Geometry check sheet. Reference: the model listing, model coordinates, mm. A direction names the side the tool comes from. Coordinates: 2 decimals unless noted, no trailing zeros. Order: outer loops, then holes, each group sorted by start corner. A loop starts at its lowest first (then second) coordinate and runs counter-clockwise, first axis right, second up. Notation, with made-up numbers: M 39.5,31 L 93.5,31 A31 ccw 93.5,56 Z; hole C 22,33.25 d7. An arc over 180 degrees is marked long. One line per item, written item: value. Start each with the question number.
1) Thickness scan on L1, parallel to X at y = 59, z = 2.5; L2, parallel to X at y = 49, z = 17; L3, parallel to X at y = -18, z = 11.5. Record the ranges inside material, lowest first. Write a range as from..to.
2) Sectioned sample at B-B, the plane x = -41.5. Enter the section's corners in (y, z), then the cut area to 3 significant figures.
3) Access from +Z, -Z, +X, -X, +Y, -Y to the whole of each face (thin tool, end or side, straight path). Record for faces 4 (the flat face through (-35.057, -29.095, 12.522)), 5 (the flat face through (53.315, 29.328, 12.522)).
4) Sectioned sample at D-D, the plane y = 75. Enter the section's corners in (x, z).
5) Go/stop test with flat-tipped pins: P1, Ø3, axis at x = -68, z = 13, coming from the +Y side; P2, Ø10, axis at y = 33.5, z = 3, coming from the +X side; P3, Ø3, axis at x = 53.5, z = 10.5, coming from the -Y side. Record where each tip stops, or that it passes through.
6) Sectioned sample at C-C, the plane z = 21.25. Enter the section's corners in (x, y), then the cut area to 3 significant figures.
7) Sectioned sample at A-A, the plane y = 35.5. Enter the section's corners in (x, z), then the cut area to 3 significant figures.
8) Draft check along Y on faces 1 (the flat face through (-25, -9, 0)), 2 (the flat face through (-52.056, 31.509, 12.522)), 3 (the flat face through (42.725, -15.813, 12.522)). Enter one of: pulls with the +Y half, pulls with the -Y half, needs draft (parallel to the pull), parting line crosses it, or undercut.
```python
from build123d import *

# Parameters (mm, degrees)
F1_DEPTH = 25.4


with BuildPart() as f1:
    # F0 (on Top) → F1 (new body)
    with BuildSketch(Plane.XY):
        Polygon((-105.146734, -61.205373), (105.578775, -60.457056), (-0.432041, 121.66243), align=None)
        Polygon((62.332636, -31.189396), (66.488145, -38.386948), (58.177127, -38.386948), (49.866109, -38.386948), (33.244072, -38.386948), (0, -38.386948), (-33.244072, -38.386948), (-49.866109, -38.386948), (-58.177127, -38.386948), (-66.488145, -38.386948), (-62.332636, -31.189396), (-58.177127, -23.991843), (-49.866109, -9.596737), (-33.244072, 19.193474), (-16.622036, 47.983686), (-8.311018, 62.378791), (-4.155509, 69.576344), (0, 76.773897), (4.155509, 69.576344), (8.311018, 62.378791), (16.622036, 47.983686), (33.244072, 19.193474), (49.866109, -9.596737), (58.177127, -23.991843), align=None, mode=Mode.SUBTRACT)
        Polygon((-58.177127, -38.386948), (-11.280757, -19.538844), (-22.561514, 0), (-62.332636, -31.189396), (-66.488145, -38.386948), align=None)
        Polygon((0, 19.538844), (11.280757, 19.538844), (4.155509, 69.576344), (0, 76.773897), (-4.155509, 69.576344), (-11.280757, 19.538844), align=None)
        Polygon((58.177127, -38.386948), (66.488145, -38.386948), (62.332636, -31.189396), (22.561514, 0), (11.280757, -19.538844), align=None)
    extrude(amount=F1_DEPTH)


solid = f1.part
```
Final values:
1. L1: x = -36.31..-10.26, -5.66..5.66, 10.26..36.04
1. L2: x = -42.04..-16.04, -7.09..7.09, 16.04..41.86
1. L3: x = -80.41..-54.72, -45.51..-12.17, 12.17..45.51, 54.72..80.86
2. outline: M -60.98,0 L -38.39,0 L -38.39,25.4 L -60.98,25.4 Z; M -31.68,0 L -14.85,0 L -14.85,25.4 L -31.68,25.4 Z; M 4.89,0 L 49.94,0 L 49.94,25.4 L 4.89,25.4 Z
2. area: 2,150 mm^2
3. face 4: +Z, -Z
3. face 5: +Z, -Z, +X, +Y
4. outline: M -27.15,0 L 26.73,0 L 26.73,25.4 L -27.15,25.4 Z
5. P1: stops at y = 6.29
5. P2: stops at x = 53.8
5. P3: stops at y = -60.65
6. outline: M -105.15,-61.21 L 105.58,-60.46 L -0.43,121.66 Z; hole M -62.33,-31.19 L -22.56,0 L -11.28,-19.54 L -58.18,-38.39 L 58.18,-38.39 L 11.28,-19.54 L 22.56,0 L 62.33,-31.19 L 4.16,69.58 L 11.28,19.54 L -11.28,19.54 L -4.16,69.58 Z
6. area: 14,000 mm^2
7. outline: M -49.77,0 L -23.83,0 L -23.83,25.4 L -49.77,25.4 Z; M -9.01,0 L 9.01,0 L 9.01,25.4 L -9.01,25.4 Z; M 23.83,0 L 49.72,0 L 49.72,25.4 L 23.83,25.4 Z
7. area: 1,770 mm^2
8. face 1: needs draft
8. face 2: pulls with the +Y half
8. face 3: undercut
